Check sheet for the drawn part. Datum: minimum x, y, z corner. Units: mm. A direction names the side the tool comes from. Give positions to 0.01 mm unless a question says otherwise; leave off trailing zeros. Write each loop counter-clockwise with the first axis right and the second up, starting at its lowest first coordinate (ties: lowest second). Pieces come first, ordered by that corner, then holes. Notation, with made-up numbers: M 46,28 L 96,28 A22 cw 96,60 Z; hole C 10,67 d9. An arc over 180 degrees is marked long. Use CSV: the item, a comma, the result in double quotes. Start each with the question number.
1. Scan lines: line 1 (Z direction, x = 133, y = 16.5); line 2 (X direction, y = 6.5, z = 133). Record each from-to range of solid material in increasing order.
2. Access from +Z, -Z, +X, -X, +Y, -Y to the whole of each face (thin tool, end or side, straight path). Record for the marked faces 4 and 5.
3. Cross-section at D-D, the plane z = 28.5. Enter the section's corners in (x, y).
4. Cross-section at A-A, the plane y = 13. Enter the section's corners in (x, z).
5. Mould release check, pull along Z, two halves, no side actions. Record for the marked faces 1, 2 and 3: +Z half, -Z half, draft (parallel to the pull), parting line (faces both ways), or undercut.
6. Cross-section at C-C, the plane y = 28. Enter the section's corners in (x, z), and give its area (3 significant figures).
7. Cross-section at B-B, the plane x = 12.5. State how many separate pieces and enclosed holes the cut face has, and give its area (3 significant figures).
8. Depth check by flat-ended pin: P1, Ø25, axis at x = 17, z = 17, coming from the +Y side; P2, Ø12, axis at x = 49.5, z = 20, coming from the +Y side. Enter the tip coordinate at first touch or a pass-through.
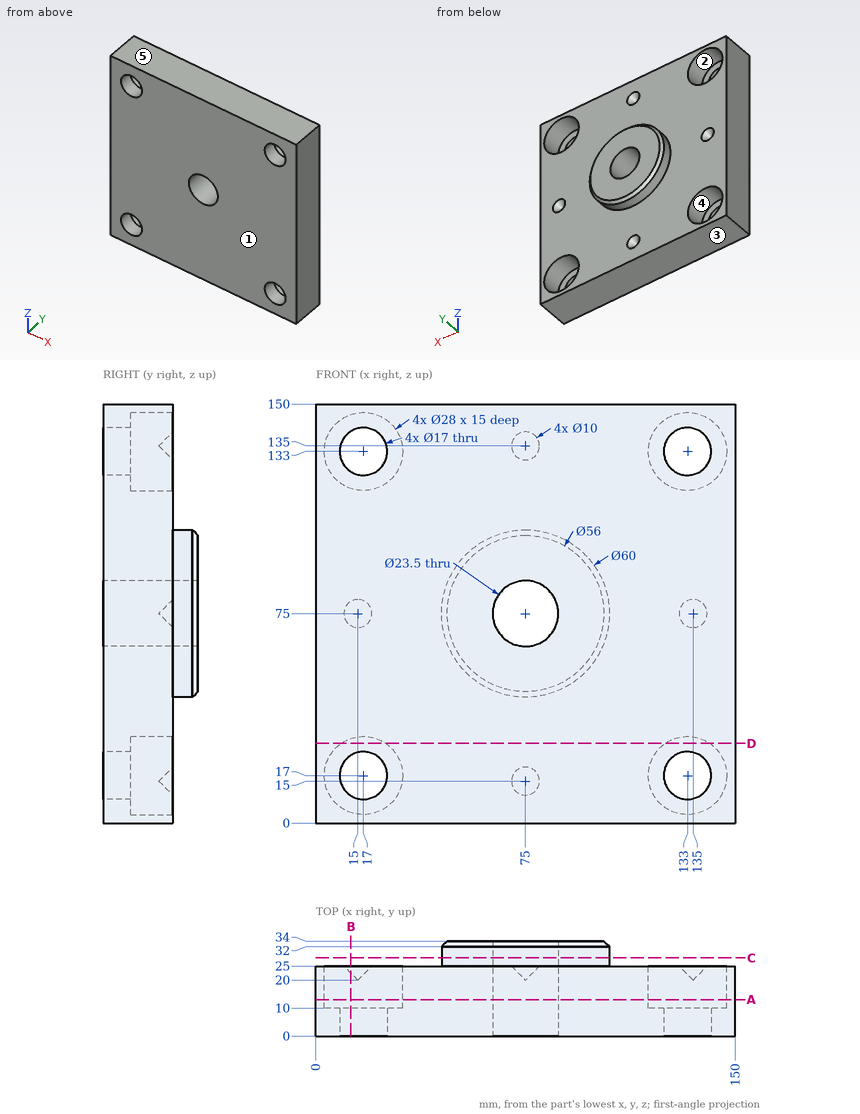
Worked answers:
1,line 1,"z = 0 to 3, 31 to 119, 147 to 150"
1,line 2,"x = 0 to 8.5, 25.5 to 124.5, 141.5 to 150"
2,face 4,"+Y"
2,face 5,"+Z, +X, -X, +Y, -Y"
3,outline,"M 0,0 L 150,0 L 150,25 L 140.98,25 L 140.98,10 L 125.02,10 L 125.02,25 L 24.98,25 L 24.98,10 L 9.02,10 L 9.02,25 L 0,25 Z"
4,outline,"M 0,0 L 150,0 L 150,150 L 0,150 Z; hole C 17,17 d28; hole C 17,133 d28; hole C 75,75 d23.5; hole C 133,17 d28; hole C 133,133 d28"
5,face 1,"draft"
5,face 2,"undercut"
5,face 3,"-Z half"
6,outline,"C 75,75 d60; hole C 75,75 d23.5"
6,area,"2,390 mm^2"
7,separate pieces,"3"
7,enclosed holes,"0"
7,area,"2,650 mm^2"
8,P1,"stops at y = 10"
8,P2,"stops at y = 25"
